The model under review builds one solid part; all positions refer to its coordinate system, in mm. Face numbers are marked on the shaded views. A direction names the side the tool comes from. Coordinates: 2 decimals unless noted, no trailing zeros. Write each loop counter-clockwise with the first axis right and the second up, starting at its lowest first coordinate (ties: lowest second). Pieces come first, ordered by that corner, then holes. Notation, with made-up numbers: M 59.5,-8.5 L 68.5,-8.5 A27 cw 68.5,28.5 Z; hole C -16,-30 d7. An arc over 180 degrees is marked long. Answer as a JSON object with one key per item and string values.
```python
from build123d import *

# Parameters (mm, degrees)
EXTRUDE_1_DEPTH          = 20
SKETCH_3_W               = 10
SKETCH_3_H               = 30
EXTRUDE_2_DEPTH          = 30
SKETCH_5_W               = 40
SKETCH_5_H               = 10
EXTRUDE_3_DEPTH          = 30
SKETCH_2_R               = 5
CUT_EXTRUDE_1_DEPTH      = 13
CUT_EXTRUDE_2_REACH      = 12
SKETCH_4_R               = 5
CUT_EXTRUDE_3_REACH      = 34
SKETCH_6_R               = 5
SKETCH_7_R               = 9
SKETCH_7_R_2             = 5
EXTRUDE_4_DEPTH          = 2
SKETCH_8_R               = 9
SKETCH_8_R_2             = 5
EXTRUDE_5_DEPTH          = 2
SKETCH_9_R               = 9
SKETCH_9_R_2             = 5
EXTRUDE_6_DEPTH          = 2
SKETCH_11_W              = 40
SKETCH_11_H              = 16
EXTRUDE_7_DEPTH          = 57
SKETCH_12_W              = 20
SKETCH_12_H              = 16
REVOLVE_1_ANGLE          = 180
SKETCH_13_R              = 15
CUT_EXTRUDE_5_DEPTH      = 35
CUT_EXTRUDE_5_DEPTH_BACK = 3
CUT_EXTRUDE_6_REACH      = 101
SKETCH_14_R              = 13
SKETCH_15_R              = 3
CUT_EXTRUDE_7_DEPTH      = 12
SKETCH_10_R              = 4
CUT_EXTRUDE_4_DEPTH      = 21
EXTRUDE_8_DEPTH          = 40
SKETCH_17_W              = 10
SKETCH_17_H              = 21
CUT_EXTRUDE_8_DEPTH      = 15
SKETCH_18_R              = 2
CUT_EXTRUDE_9_DEPTH      = 40
SKETCH_19_W              = 30
SKETCH_19_H              = 10
EXTRUDE_9_DEPTH          = 32
SKETCH_20_R              = 3
CUT_EXTRUDE_10_DEPTH     = 20
SKETCH_21_W              = 35
SKETCH_21_H              = 20
EXTRUDE_10_DEPTH         = 40
SKETCH_22_W              = 35
SKETCH_22_H              = 20
EXTRUDE_11_DEPTH         = 140


with BuildPart() as part:
    # 草图1 → 凸台-拉伸1 (new body)
    with BuildSketch(Plane(origin=(0, 0, 0), x_dir=(1, 0, 0), z_dir=(0, 1, 0))):
        Polygon((-67, 0), (67, 0), (67, 22), (107, 22), (107, 42), (143.5, 42), (143.5, 116), (72, 116), (72, 96), (12, 96), (12, 136), (-12, 136), (-12, 96), (-72, 96), (-72, 116), (-143.5, 116), (-143.5, 42), (-107, 42), (-107, 22), (-67, 22), align=None)
    extrude(amount=EXTRUDE_1_DEPTH)

    # 草图3 → 凸台-拉伸2 (add)
    with BuildSketch(Plane(origin=(0, 20, 0), x_dir=(1, 0, 0), z_dir=(0, 1, 0))):
        with Locations((-138.5, 77)):
            Rectangle(SKETCH_3_W, SKETCH_3_H)
    extrude(amount=EXTRUDE_2_DEPTH)

    # 草图5 → 凸台-拉伸3 (add)
    with BuildSketch(Plane(origin=(0, 20, 0), x_dir=(1, 0, 0), z_dir=(0, 1, 0))):
        with Locations((-87, 27)):
            Rectangle(SKETCH_5_W, SKETCH_5_H)
        with Locations((87, 27)):
            Rectangle(SKETCH_5_W, SKETCH_5_H)
    extrude(amount=EXTRUDE_3_DEPTH)

    # 草图2 → 切除-拉伸1 (cut)
    with BuildSketch(Plane(origin=(0, 20, 0), x_dir=(1, 0, 0), z_dir=(0, 1, 0))):
        with Locations((0, 93)):
            Circle(SKETCH_2_R)
        with Locations((-41, 46)):
            Circle(SKETCH_2_R)
        with Locations((41, 46)):
            Circle(SKETCH_2_R)
    extrude(amount=-CUT_EXTRUDE_1_DEPTH, mode=Mode.SUBTRACT)

    # 草图4 → 切除-拉伸2 (cut, up to next)
    with BuildSketch(Plane(origin=(-133.5, 0, 0), x_dir=(0, 0, -1), z_dir=(1, 0, 0)), mode=Mode.PRIVATE) as cut_extrude_2_sk1:
        with Locations((77, 38)):
            Circle(SKETCH_4_R)
    cut_extrude_2_tool1 = extrude(cut_extrude_2_sk1.sketch, amount=-CUT_EXTRUDE_2_REACH, mode=Mode.PRIVATE) & part.part
    add(cut_extrude_2_tool1.solids().sort_by_distance((-133.5, 38, -77))[0], mode=Mode.SUBTRACT)

    # 草图6 → 切除-拉伸3 (cut, up to next)
    with BuildSketch(Plane(origin=(0, 0, -32), x_dir=(-1, 0, 0), z_dir=(0, 0, -1)), mode=Mode.PRIVATE) as cut_extrude_3_sk1:
        with Locations((87, 38)):
            Circle(SKETCH_6_R)
    cut_extrude_3_tool1 = extrude(cut_extrude_3_sk1.sketch, amount=-CUT_EXTRUDE_3_REACH, mode=Mode.PRIVATE) & part.part
    add(cut_extrude_3_tool1.solids().sort_by_distance((-87, 38, -32))[0], mode=Mode.SUBTRACT)
    # 草图6 → 切除-拉伸3 (cut, up to next)
    with BuildSketch(Plane(origin=(0, 0, -32), x_dir=(-1, 0, 0), z_dir=(0, 0, -1)), mode=Mode.PRIVATE) as cut_extrude_3_sk2:
        with Locations((-87, 38)):
            Circle(SKETCH_6_R)
    cut_extrude_3_tool2 = extrude(cut_extrude_3_sk2.sketch, amount=-CUT_EXTRUDE_3_REACH, mode=Mode.PRIVATE) & part.part
    add(cut_extrude_3_tool2.solids().sort_by_distance((87, 38, -32))[0], mode=Mode.SUBTRACT)

    # 草图7 → 凸台-拉伸4 (add)
    with BuildSketch(Plane(origin=(-133.5, 0, 0), x_dir=(0, 0, -1), z_dir=(1, 0, 0))):
        with Locations((77, 38)):
            Circle(SKETCH_7_R)
        with Locations((77, 38)):
            Circle(SKETCH_7_R_2, mode=Mode.SUBTRACT)
    extrude(amount=EXTRUDE_4_DEPTH)

    # 草图8 → 凸台-拉伸5 (add)
    with BuildSketch(Plane(origin=(0, 0, -32), x_dir=(-1, 0, 0), z_dir=(0, 0, -1))):
        with Locations((-87, 38)):
            Circle(SKETCH_8_R)
        with Locations((-87, 38)):
            Circle(SKETCH_8_R_2, mode=Mode.SUBTRACT)
        with Locations((87, 38)):
            Circle(SKETCH_8_R)
        with Locations((87, 38)):
            Circle(SKETCH_8_R_2, mode=Mode.SUBTRACT)
    extrude(amount=EXTRUDE_5_DEPTH)

    # 草图9 → 凸台-拉伸6 (add)
    with BuildSketch(Plane(origin=(0, 20, 0), x_dir=(1, 0, 0), z_dir=(0, 1, 0))):
        with Locations((-41, 46)):
            Circle(SKETCH_9_R)
        with Locations((-41, 46)):
            Circle(SKETCH_9_R_2, mode=Mode.SUBTRACT)
        with Locations((0, 93)):
            Circle(SKETCH_9_R)
        with Locations((0, 93)):
            Circle(SKETCH_9_R_2, mode=Mode.SUBTRACT)
        with Locations((41, 46)):
            Circle(SKETCH_9_R)
        with Locations((41, 46)):
            Circle(SKETCH_9_R_2, mode=Mode.SUBTRACT)
    extrude(amount=EXTRUDE_6_DEPTH)

    # 草图11 → 凸台-拉伸7 (add)
    with BuildSketch(Plane(origin=(0, 20, 0), x_dir=(1, 0, 0), z_dir=(0, 1, 0))):
        with Locations((0, 42)):
            Rectangle(SKETCH_11_W, SKETCH_11_H)
    extrude(amount=EXTRUDE_7_DEPTH)

    # 草图12 → 旋转1 (revolve)
    with BuildSketch(Plane(origin=(0, 77, 0), x_dir=(1, 0, 0), z_dir=(0, 1, 0))):
        with Locations((-10, 42)):
            Rectangle(SKETCH_12_W, SKETCH_12_H)
    revolve(axis=Axis((0, 77, -50), (0, 0, -1)), revolution_arc=REVOLVE_1_ANGLE)

    # 草图13 → 切除-拉伸5 (cut, two sides)
    with BuildSketch(Plane.XY.offset(-34)) as cut_extrude_5_sk:
        with Locations((0, 77)):
            Circle(SKETCH_13_R)
    extrude(amount=CUT_EXTRUDE_5_DEPTH, mode=Mode.SUBTRACT)
    extrude(cut_extrude_5_sk.sketch, amount=-CUT_EXTRUDE_5_DEPTH_BACK, mode=Mode.SUBTRACT)

    # 草图14 → 切除-拉伸6 (cut, up to next)
    with BuildSketch(Plane.XY.offset(-37), mode=Mode.PRIVATE) as cut_extrude_6_sk1:
        with Locations((0, 77)):
            Circle(SKETCH_14_R)
    cut_extrude_6_tool1 = extrude(cut_extrude_6_sk1.sketch, amount=-CUT_EXTRUDE_6_REACH, mode=Mode.PRIVATE) & part.part
    add(cut_extrude_6_tool1.solids().sort_by_distance((0, 77, -37))[0], mode=Mode.SUBTRACT)

    # 草图15 → 切除-拉伸7 (cut)
    with BuildSketch(Plane.XY.offset(-34)):
        with Locations((0, 57)):
            Circle(SKETCH_15_R)
    extrude(amount=-CUT_EXTRUDE_7_DEPTH, mode=Mode.SUBTRACT)

    # 草图10 → 切除-拉伸4 (cut, through all)
    with BuildSketch(Plane(origin=(0, 20, 0), x_dir=(1, 0, 0), z_dir=(0, 1, 0))):
        with Locations((-41, 25.75)):
            Circle(SKETCH_10_R)
        with Locations((41, 25.75)):
            Circle(SKETCH_10_R)
        with Locations((-41, 3.75)):
            Circle(SKETCH_10_R)
        with Locations((41, 3.75)):
            Circle(SKETCH_10_R)
        with Locations((-91, 69)):
            Circle(SKETCH_10_R)
        with Locations((0, 113.25)):
            Circle(SKETCH_10_R)
        with Locations((0, 135.25)):
            Circle(SKETCH_10_R)
        with Locations((85.5, 69)):
            Circle(SKETCH_10_R)
    extrude(amount=-CUT_EXTRUDE_4_DEPTH, mode=Mode.SUBTRACT)

    # 草图16 → 凸台-拉伸8 (add)
    with BuildSketch(Plane(origin=(107, 0, 0), x_dir=(0, 0, -1), z_dir=(1, 0, 0))):
        with BuildLine():
            Line((22, 50), (22, 60))
            ThreePointArc((22, 60), (27, 65), (32, 60))
            Line((32, 60), (32, 50))
            Line((32, 50), (22, 50))
        make_face()
    extrude_8 = extrude(amount=-EXTRUDE_8_DEPTH)

    # 草图17 → 切除-拉伸8 (cut)
    with BuildSketch(Plane(origin=(45, 50, 0), x_dir=(0, 0, -1), z_dir=(0, -1, 0))):
        with Locations((27, 42)):
            Rectangle(SKETCH_17_W, SKETCH_17_H)
    cut_extrude_8 = extrude(amount=-CUT_EXTRUDE_8_DEPTH, mode=Mode.SUBTRACT)

    # 草图18 → 切除-拉伸9 (cut)
    with BuildSketch(Plane(origin=(107, 0, 0), x_dir=(0, 0, -1), z_dir=(1, 0, 0))):
        with Locations((27, 60)):
            Circle(SKETCH_18_R)
    cut_extrude_9 = extrude(amount=-CUT_EXTRUDE_9_DEPTH, mode=Mode.SUBTRACT)

    # 镜向1: 凸台-拉伸8, 切除-拉伸8, 切除-拉伸9 across plane
    add(extrude_8.mirror(Plane(origin=(0, 0, 0), x_dir=(0, 0, 1), z_dir=(1, 0, 0))))
    add(cut_extrude_8.mirror(Plane(origin=(0, 0, 0), x_dir=(0, 0, 1), z_dir=(1, 0, 0))), mode=Mode.SUBTRACT)
    add(cut_extrude_9.mirror(Plane(origin=(0, 0, 0), x_dir=(0, 0, 1), z_dir=(1, 0, 0))), mode=Mode.SUBTRACT)

    # 草图19 → 凸台-拉伸9 (add)
    with BuildSketch(Plane(origin=(0, 20, 0), x_dir=(1, 0, 0), z_dir=(0, 1, 0))):
        with Locations((-87, 111)):
            Rectangle(SKETCH_19_W, SKETCH_19_H)
        with Locations((87, 111)):
            Rectangle(SKETCH_19_W, SKETCH_19_H)
    extrude(amount=EXTRUDE_9_DEPTH)

    # 草图20 → 切除-拉伸10 (cut)
    with BuildSketch(Plane(origin=(0, 0, -116), x_dir=(-1, 0, 0), z_dir=(0, 0, -1))):
        with Locations((-87, 38)):
            Circle(SKETCH_20_R)
        with Locations((87, 38)):
            Circle(SKETCH_20_R)
    extrude(amount=-CUT_EXTRUDE_10_DEPTH, mode=Mode.SUBTRACT)

    # 草图21 → 凸台-拉伸10 (add)
    with BuildSketch(Plane(origin=(0, 0, -116), x_dir=(-1, 0, 0), z_dir=(0, 0, -1))):
        with Locations((-126, 10)):
            Rectangle(SKETCH_21_W, SKETCH_21_H)
        with Locations((126, 10)):
            Rectangle(SKETCH_21_W, SKETCH_21_H)
    extrude(amount=EXTRUDE_10_DEPTH)

    # 草图22 → 凸台-拉伸11 (add)
    with BuildSketch(Plane(origin=(0, 20, 0), x_dir=(1, 0, 0), z_dir=(0, 1, 0))):
        with Locations((-126, 146)):
            Rectangle(SKETCH_22_W, SKETCH_22_H)
        with Locations((126, 146)):
            Rectangle(SKETCH_22_W, SKETCH_22_H)
    extrude(amount=EXTRUDE_11_DEPTH)


solid = part.part
```
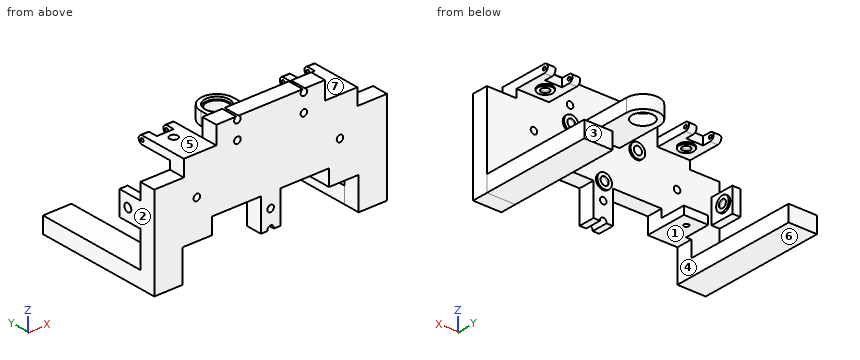
(1) For the marked faces 4, 5, 6 and 7, list the 3-axis set-ups (+Z, -Z, +X, -X, +Y, -Y) from which the entire face can be reached by the end or side of a thin tool; tool diameter is ignored.
Results list:
{"face 4": "-Z, +Y, -Y", "face 5": "+Z, -X, +Y, -Y", "face 6": "-Z, +X, -X, +Y, -Y", "face 7": "+Z, +X, +Y, -Y"}
(2) Wall thickness on line 1 along X through (y, z) = (6, -135.25); line 2 along Z through (x, y) = (85.5, 12.5); line 3 along Y through (x, z) = (-103.25, -27): over which ranges is each line inside the solid? List them lowest first. Write a range as from..to.
Results list:
{"line 1": "-143.5..-108.5, -12..-4, 4..12, 108.5..143.5", "line 2": "-116..-73, -65..-22", "line 3": "0..58, 62..65"}
(3) Add section D-D on z = -16. Give the boundary of the cut face in (x, y), and give its area (3 significant figures).
Results list:
{"outline": "M -67,0 L 67,0 L 67,20 L -67,20 Z", "area": "2,680 mm²"}
(4) Add section B-B on y = 104. Give the boundary of the cut face in (x, z).
Results list:
{"outline": "M -143.5,-156 L -108.5,-156 L -108.5,-136 L -143.5,-136 Z; M 108.5,-156 L 143.5,-156 L 143.5,-136 L 108.5,-136 Z"}
(5) Draft analysis for pull direction X (two halves, no side actions). For the marked faces 1, 2 and 3, state which applies: released by +X, released by -X, zero draft, split by the parting line, or undercut.
Results list:
{"face 1": "undercut", "face 2": "released by -X", "face 3": "zero draft"}
(6) Add section C-C on y = 69. Give the boundary of the cut face in (x, z).
Results list:
{"outline": "M -143.5,-156 L -108.5,-156 L -108.5,-136 L -143.5,-136 Z; M -20,-50 L -10.25,-50 L -10.25,-37 L -12.69,-37 L -12.69,-34 L -20,-34 Z; M 10.25,-50 L 20,-50 L 20,-34 L 12.69,-34 L 12.69,-37 L 10.25,-37 Z; M 108.5,-156 L 143.5,-156 L 143.5,-136 L 108.5,-136 Z"}
(7) For pin 1 Ø9 at (x, y) = (87, 38) entering from -Z; pin 2 Ø10.5 at (x, z) = (-41, -25.75) entering from +Y; pin 3 Ø4.5 at (y, z) = (60, -27) entering from +X; pin 4 Ø5 at (y, z) = (135, -131.5) entering from +X, all flat-tipped, find the tip position at first contact; note any pin that passes through.
Results list:
{"pin 1": "z = -116", "pin 2": "y = 20", "pin 3": "x = 107", "pin 4": "through"}
(8) Add section A-A on z = -77. Give the boundary of the cut face in (x, y).
Results list:
{"outline": "M -143.5,0 L 143.5,0 L 143.5,20 L -133.5,20 L -133.5,29 L -131.5,29 L -131.5,33 L -143.5,33 Z; M -143.5,43 L -131.5,43 L -131.5,47 L -133.5,47 L -133.5,50 L -143.5,50 Z"}
